Can you work these out from the model? Positions are in its coordinate system, mm. Face numbers are marked on the shaded views. Give positions to 0.01 mm unless a question says otherwise; leave off trailing zeros. Loops run counter-clockwise (first coordinate to the right, second up) from the corner with the lowest first, then second, coordinate; pieces in that order, holes last. Notation, with made-up numbers: (-26.75, 13.5) - (-1.75, 13.5) arc R13 ccw to (-1.75, 30.5) - close; hole circle Ø7 at (-27, -27.75). An arc over 180 degrees is marked (long way). Answer in a Markdown table with one row per item.
from build123d import *

# Parameters (mm, degrees)
SKETCH_1_W          = 28
SKETCH_1_H          = 15
SKETCH_1_R          = 3.25
EXTRUDE_1_DEPTH     = 7.5
SKETCH_2_R          = 2.2
CUT_EXTRUDE_1_DEPTH = 15
FILLET_1_R          = 1
CHAMFER_1_SIZE      = 1


with BuildPart() as part:
    # 草图1 → 凸台-拉伸1 (new, symmetric)
    with BuildSketch(Plane(origin=(0, 0, 0), x_dir=(1, 0, 0), z_dir=(0, 1, 0))):
        Rectangle(SKETCH_1_W, SKETCH_1_H)
        with Locations(Location((0, 0, 0), (0, 0, 270))):
            Circle(SKETCH_1_R, mode=Mode.SUBTRACT)
    extrude(amount=EXTRUDE_1_DEPTH, both=True)

    # 草图2 → 切除-拉伸1 (cut)
    with BuildSketch(Plane.XY.offset(7.5)):
        with Locations((-10, 0)):
            Circle(SKETCH_2_R)
        with Locations((10, 0)):
            Circle(SKETCH_2_R)
    extrude(amount=-CUT_EXTRUDE_1_DEPTH, mode=Mode.SUBTRACT)

    # 圆角1
    fillet_1_edges = [part.edges().sort_by_distance(p)[0] for p in [
        (-14, 7.5, 0),
        (0, 7.5, 7.5),
        (14, 7.5, 0),
        (0, -7.5, 7.5),
        (-14, -7.5, 0),
        (0, -7.5, -7.5),
        (14, -7.5, 0),
        (14, 0, 7.5),
        (-14, 0, 7.5),
        (-14, 0, -7.5),
        (14, 0, -7.5),
        (0, 7.5, -7.5),
    ]]
    fillet(fillet_1_edges, radius=FILLET_1_R)

    # 倒角1
    chamfer_1_edges = [part.edges().sort_by_distance(p)[0] for p in [
        (0, -7.5, -3.25),
        (0, 7.5, -3.25),
    ]]
    chamfer(chamfer_1_edges, length=CHAMFER_1_SIZE)


solid = part.part
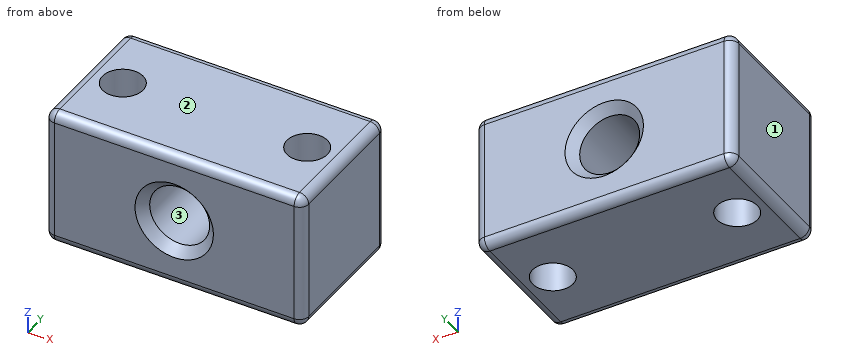
Q1. Imagine slicing it at C-C, the plane x = 0. Write out the boundary of the cut face in (y, z), and give its area (3 significant figures).
Checked values:
| item | result |
|---|---|
| outline | (-7.5, -6.5) arc R1 ccw to (-6.5, -7.5) - (6.5, -7.5) arc R1 ccw to (7.5, -6.5) - (7.5, -4.25) - (6.5, -3.25) - (-6.5, -3.25) - (-7.5, -4.25) - close; (-7.5, 4.25) - (-6.5, 3.25) - (6.5, 3.25) - (7.5, 4.25) - (7.5, 6.5) arc R1 ccw to (6.5, 7.5) - (-6.5, 7.5) arc R1 ccw to (-7.5, 6.5) - close |
| area | 125 mm² |
Q2. Imagine slicing it at D-D, the plane y = 2.75. Write out the boundary of the cut face in (x, z), and give its area (3 significant figures).
Checked values:
| item | result |
|---|---|
| outline | (-14, -6.5) arc R1 ccw to (-13, -7.5) - (13, -7.5) arc R1 ccw to (14, -6.5) - (14, 6.5) arc R1 ccw to (13, 7.5) - (-13, 7.5) arc R1 ccw to (-14, 6.5) - close; hole circle Ø6.5 at (0, 0) |
| area | 386 mm² |
Q3. If I drill on line 1 (Y direction, x = -10, z = 3.5); line 2 (X direction, y = -1, z = -0.5); line 3 (X direction, y = 1, z = 3.75), over which ranges is the centre line in solid material (lowest first)? Write a range as [from, to].
Checked values:
| item | result |
|---|---|
| line 1 | y = [-7.5, -2.2], [2.2, 7.5] |
| line 2 | x = [-14, -11.96], [-8.04, -3.21], [3.21, 8.04], [11.96, 14] |
| line 3 | x = [-14, -11.96], [-8.04, 8.04], [11.96, 14] |
Q4. Imagine slicing it at A-A, the plane z = 0. Write out the boundary of the cut face in (x, y).
Checked values:
| item | result |
|---|---|
| outline | (-14, -6.5) arc R1 ccw to (-13, -7.5) - (-4.25, -7.5) - (-3.25, -6.5) - (-3.25, 6.5) - (-4.25, 7.5) - (-13, 7.5) arc R1 ccw to (-14, 6.5) - close; (3.25, -6.5) - (4.25, -7.5) - (13, -7.5) arc R1 ccw to (14, -6.5) - (14, 6.5) arc R1 ccw to (13, 7.5) - (4.25, 7.5) - (3.25, 6.5) - close; hole circle Ø4.4 at (-10, 0); hole circle Ø4.4 at (10, 0) |
Q5. Imagine slicing it at B-B, the plane y = 0. Write out the boundary of the cut face in (x, z).
Checked values:
| item | result |
|---|---|
| outline | (-14, -6.5) arc R1 ccw to (-13, -7.5) - (-12.2, -7.5) - (-12.2, 7.5) - (-13, 7.5) arc R1 ccw to (-14, 6.5) - close; (-7.8, -7.5) - (7.8, -7.5) - (7.8, 7.5) - (-7.8, 7.5) - close; (12.2, -7.5) - (13, -7.5) arc R1 ccw to (14, -6.5) - (14, 6.5) arc R1 ccw to (13, 7.5) - (12.2, 7.5) - close; hole circle Ø6.5 at (0, 0) |
Q6. If we mould it in two halves opening along Z, with no side actions, what happens to the marked faces 1, 2 and 3? For each: released by +Z, released by -Z, zero draft, split by the parting line, or undercut.
Checked values:
| item | result |
|---|---|
| face 1 | zero draft |
| face 2 | released by +Z |
| face 3 | undercut |
